```python
from build123d import *

# Parameters (mm, degrees)
CUT_EXTRUDE1_DEPTH = 0.9


with BuildPart() as part:
    # Sketch1 → Revolve1 (revolve)
    with BuildSketch(Plane.XY):
        with BuildLine():
            Line((0, 0), (0, 1.001109878))
            ThreePointArc((0, 1.001109878), (0.459937132, 2.081974916), (1.557692308, 2.5))
            ThreePointArc((1.557692308, 2.5), (1.694115338, 2.438823033), (1.75, 2.300147984))
            Line((1.75, 2.300147984), (1.75, 1.7))
            ThreePointArc((1.75, 1.7), (1.808578644, 1.558578644), (1.95, 1.5))
            Line((1.95, 1.5), (7.4, 1.5))
            Line((7.4, 1.5), (7.75, 1.15))
            Line((7.75, 1.15), (7.75, 0))
            Line((7.75, 0), (0, 0))
        make_face()
    revolve(axis=Axis((0, 0, 0), (-1, 0, 0)))

    # Sketch2 → Cut-Extrude1 (cut)
    with BuildSketch(Plane.ZY):
        Polygon((1, -0.577350269), (1, 0.577350269), (0, 1.154700538), (-1, 0.577350269), (-1, -0.577350269), (0, -1.154700538), align=None)
    extrude(amount=-CUT_EXTRUDE1_DEPTH, mode=Mode.SUBTRACT)


solid = part.part
```
Geometry check sheet. Reference: the model listing, model coordinates, mm. A direction names the side the tool comes from. Coordinates: 2 decimals unless noted, no trailing zeros. Order: outer loops, then holes, each group sorted by start corner. A loop starts at its lowest first (then second) coordinate and runs counter-clockwise, first axis right, second up.
Q1. Depth check by flat-ended pin: pin 1 Ø0.7 at (x, y) = (0.5, 0) entering from +Z; pin 2 Ø0.5 at (x, y) = (0.5, 0) entering from -Z; pin 3 Ø3 at (x, z) = (5, 0.5) entering from -Y. Enter the tip coordinate at first touch or a pass-through.
Reply:
pin 1: stops at z = 2.35
pin 2: stops at z = -2.3
pin 3: stops at y = -1.5
Q2. Tool access check on faces 4 (the face through (1.75, 0, 2)), 5 (the face through (0.44, -0.87, 0.49)). Record the directions out of +Z, -Z, +X, -X, +Y, -Y that give a thin tool (end or side, any length) a straight path to the whole face; none if there is none.
Reply:
face 4: +X
face 5: -X
Q3. Sectioned sample at A-A on x = 5.75. Record the cut outline in (y, z), and give its area (3 significant figures).
Reply:
outline: circle Ø3 at (0, 0)
area: 7.07 mm2
Q4. Draft check along Z on faces 1 (the face through (0.4, 0, -1)), 2 (the face through (4.71, -1.5, -0.07)), 3 (the face through (7.75, 0, 0)). Enter one of: released by +Z, released by -Z, zero draft, split by the parting line, or undercut.
Reply:
face 1: undercut
face 2: split by the parting line
face 3: zero draft
Q5. Thickness scan on probe 1 along X at (y, z) = (0.05, -0.2); probe 2 along Z at (x, y) = (3.5, -0.3); probe 3 along Z at (x, y) = (0.5, 0.8). Record the ranges inside material, lowest first.
Reply:
probe 1: x = 0.9 to 7.75
probe 2: z = -1.47 to 1.47
probe 3: z = -1.96 to -0.61, 0.61 to 1.96
